For this review, take the finished solid that the model builds, in its own axes (mm). Coordinates: 2 decimals unless noted, no trailing zeros. Loops run counter-clockwise (first coordinate to the right, second up) from the corner with the lowest first, then second, coordinate; pieces in that order, holes last. Notation, with made-up numbers: M 57,-38 L 98,-38 A29 cw 98,-16 Z; hole C -5.5,48 d3. An arc over 180 degrees is marked long. Use one line per item in the form item = value.
Autodesk Inventor part; units mm, degrees
ref_plane "YZ Plane" through (0, 0, 0) normal (1, 0, 0) x (0, 1, 0)
ref_plane "XZ Plane" through (0, 0, 0) normal (0, 1, 0) x (-1, 0, 0)
ref_plane "XY Plane" through (0, 0, 0) normal (0, 0, 1) x (1, 0, 0)
sketch "Sketch1" plane through (0, 0, 0) normal (0, 0, 1) x (1, 0, 0)
  line L0 (152.4, -209.55) -> (-152.4, -209.55)
  line L1 (-152.4, -209.55) -> (-152.4, 209.55)
  line L2 (-152.4, 209.55) -> (152.4, 209.55)
  line L3 (152.4, 209.55) -> (152.4, -209.55)
  line L4 (152.4, -209.55) -> (-152.4, 209.55) construction
  line L5 (-152.4, -209.55) -> (152.4, 209.55) construction
  line L6 (57.6, 93.25) -> (57.6, -93.25) construction
  point P0 (0, 0)
  point P1 (57.6, 55.75)
  point P2 (57.6, -55.75)
  point P3 (57.6, 0)
  point P4 (152.4, 0)
  dimension "d0" = 304.8
  dimension "d1" = 419.1
  dimension "d2" = 111.5
  dimension "d3" = 37.5
  dimension "d4" = 37.5
  dimension "d25" = 210
extrude "Extrusion1" add sketch "Sketch1" against normal blind 5.588
hole "Hole1" at (57.6, 55.75, 0) at (57.6, -55.75, 0) at (57.6, -93.25, 0) at (57.6, 93.25, 0) direction (0, 0, -1) diameter 7.1437 end through all
sketch "Sketch2" plane through (0, 0, 0) normal (0, 0, 1) x (1, 0, 0)
  line L0 (-127.4, 74.5) -> (7.6, 74.5) construction
  line L1 (-127.4, -74.5) -> (7.6, -74.5) construction
  circle A0 centre (57.6, 55.75) radius 3.5719 construction
  circle A1 centre (57.6, -55.75) radius 3.5719
  circle A2 centre (57.6, 93.25) radius 3.5719 construction
  line L2 (57.6, 93.25) -> (57.6, 55.75) construction
  circle A3 centre (57.6, -93.25) radius 3.5719 construction
  line L3 (57.6, -93.25) -> (57.6, -55.75) construction
  point P0 (0, 0)
  point P1 (57.6, -74.5)
  point P2 (57.6, 74.5)
  dimension "d15" = 50
  dimension "d16" = 50
  dimension "d17" = 135
hole "Hole2" at (-127.4, 74.5, 0) at (7.6, 74.5, 0) at (7.6, -74.5, 0) at (-127.4, -74.5, 0) direction (0, 0, -1) diameter 7.1437 end through all
sketch "Sketch3" plane through (0, 0, 0) normal (0, 0, 1) x (1, 0, 0)
  line L0 (12.7, -193.675) -> (-12.7, -193.675) construction
  line L1 (-12.7, -193.675) -> (-12.7, -136.525) construction
  line L2 (-12.7, -136.525) -> (12.7, -136.525) construction
  line L3 (12.7, -136.525) -> (12.7, -193.675) construction
  line L4 (12.7, -193.675) -> (-12.7, -136.525) construction
  line L5 (-12.7, -193.675) -> (12.7, -136.525) construction
  line L6 (-12.7, 136.525) -> (12.7, 136.525) construction
  line L7 (12.7, 136.525) -> (12.7, 193.675) construction
  line L8 (12.7, 193.675) -> (-12.7, 193.675) construction
  line L9 (-12.7, 193.675) -> (-12.7, 136.525) construction
  line L10 (-12.7, 136.525) -> (12.7, 193.675) construction
  line L11 (12.7, 136.525) -> (-12.7, 193.675) construction
  line L12 (-23.8125, -202.4062) -> (23.8125, -202.4062) construction
  line L13 (23.8125, -202.4062) -> (23.8125, -127.7938) construction
  line L14 (23.8125, -127.7938) -> (-23.8125, -127.7938) construction
  line L15 (-23.8125, -127.7938) -> (-23.8125, -202.4062) construction
  line L16 (-23.8125, -202.4062) -> (23.8125, -127.7938) construction
  line L17 (23.8125, -202.4062) -> (-23.8125, -127.7938) construction
  line L18 (-23.8125, 127.7938) -> (23.8125, 127.7938) construction
  line L19 (23.8125, 127.7938) -> (23.8125, 202.4062) construction
  line L20 (23.8125, 202.4062) -> (-23.8125, 202.4062) construction
  line L21 (-23.8125, 202.4062) -> (-23.8125, 127.7938) construction
  line L22 (-23.8125, 127.7938) -> (23.8125, 202.4062) construction
  line L23 (23.8125, 127.7938) -> (-23.8125, 202.4062) construction
  line L24 (0, -165.1) -> (0, 165.1) construction
  line L25 (-152.4, -209.55) -> (152.4, -209.55) construction
  point P0 (0, 0)
  point P1 (0, 0)
  dimension "d26" = 25.4
  dimension "d27" = 57.15
  dimension "d28" = 25.4
  dimension "d29" = 57.15
  dimension "d30" = 47.625
  dimension "d31" = 74.6125
  dimension "d33" = 330.2
hole "Hole3" at (12.7, 193.675, 0) at (12.7, 136.525, 0) at (-12.7, 136.525, 0) at (-12.7, 193.675, 0) at (12.7, -136.525, 0) at (12.7, -193.675, 0) at (-12.7, -193.675, 0) at (-12.7, -136.525, 0) direction (0, 0, -1) diameter 8.7313 end through all
properties part number "Base Plate" material "Polycarbonate, Clear"
1. For pin 1 Ø5.5 at (x, y) = (57.6, -93.25) entering from +Z, flat-tipped, find the tip position at first contact; note if it passes through.
Computed values:
pin_1 = through
2. Wall thickness on line 1 along Y through (x, z) = (-12.7, -1.85); line 2 along Y through (x, z) = (57.6, -1.85); line 3 along X through (y, z) = (74.5, -1.85): over which ranges is each line inside the solid? List them lowest first. Write a range as from..to.
Computed values:
line_1 = -209.55..-198.04, -189.31..-140.89, -132.16..132.16, 140.89..189.31, 198.04..209.55
line_2 = -209.55..-96.82, -89.68..-59.32, -52.18..52.18, 59.32..89.68, 96.82..209.55
line_3 = -152.4..-130.97, -123.83..4.03, 11.17..152.4
3. Draft analysis for pull direction Y (two halves, no side actions). For faces 1 (the face through (9.019, -196.022, -2.833)), 2 (the face through (-2, 3, -5.588)), 3 (the face through (14.37, 189.64, -2.83)), state which applies: +Y half, -Y half, draft (parallel to the pull), parting line (faces both ways), or undercut.
Computed values:
face_1 = undercut
face_2 = draft
face_3 = undercut
4. Consider section A-A on x = -12.7. Write out the cut boundary in (y, z).
Computed values:
outline = M -209.55,-5.59 L -198.04,-5.59 L -198.04,0 L -209.55,0 Z; M -189.31,-5.59 L -140.89,-5.59 L -140.89,0 L -189.31,0 Z; M -132.16,-5.59 L 132.16,-5.59 L 132.16,0 L -132.16,0 Z; M 140.89,-5.59 L 189.31,-5.59 L 189.31,0 L 140.89,0 Z; M 198.04,-5.59 L 209.55,-5.59 L 209.55,0 L 198.04,0 Z
